Autodesk Inventor part; units mm, degrees
ref_plane "Work Plane1" through (0, -40, 0) normal (-1, 0, 0) x (0, 0, 1)
ref_plane "Work Plane2" through (-196.6667, -40, 18) normal (1, 0, 0) x (0, 0, -1)
ref_plane "YZ Plane" through (0, 0, 0) normal (1, 0, 0) x (0, 1, 0)
sketch "Sketch1" plane through (0, 0, 0) normal (0, 0, 1) x (1, 0, 0)
  line L0 (-590, 40) -> (590, 40)
  line L1 (590, 40) -> (590, -40)
  line L2 (590, -40) -> (-590, -40)
  line L3 (-590, -40) -> (-590, 40)
  point P0 (0, 0)
  point P1 (-590, 0)
  point P2 (0, 40)
  dimension "d0" = 80
  dimension "d1" = 1180
extrude "Extrusion1" add sketch "Sketch1" along normal blind 18
sketch "Sketch2" plane through (0, 0, 18) normal (0, 0, 1) x (1, 0, 0)
  line L0 (590, 40) -> (-590, 40)
  line L1 (-590, 40) -> (-590, -40)
  line L2 (-590, -40) -> (590, -40)
  line L3 (590, -40) -> (590, 40)
  line L4 (-590, 58) -> (-531, 58)
  line L5 (-531, 58) -> (-531, 40)
  line L6 (-531, 40) -> (-590, 40)
  line L7 (-590, 40) -> (-590, 58)
  point P0 (0, 0)
  point P1 (-560.5, 40)
  point P2 (0, 40)
  point P3 (-590, 49)
  point P4 (-590, 0)
  dimension "d4" = 18
  dimension "d5" = 59
extrude "Extrusion2" add sketch "Sketch2" against normal blind 18 contours L0 L7 L4 L5
ref_plane "Work Plane1" through (0, -40, 0) normal (-1, 0, 0) x (0, 0, 1)
sketch "Sketch3" plane through (0, 0, 18) normal (0, 0, 1) x (1, 0, 0)
  line L0 (-246.6667, 58) -> (-146.6667, 58)
  line L1 (-146.6667, 58) -> (-146.6667, 40)
  line L2 (-146.6667, 40) -> (-246.6667, 40)
  line L3 (-246.6667, 40) -> (-246.6667, 58)
  line L4 (590, 40) -> (-531, 40)
  line L5 (-531, 58) -> (-531, 40)
  line L6 (-590, 58) -> (-531, 58)
  line L7 (-590, -40) -> (-590, 58)
  line L8 (-590, -40) -> (590, -40)
  line L9 (590, -40) -> (590, 40)
  point P0 (0, 0)
  point P1 (-196.6667, 40)
  point P2 (29.5, 40)
  dimension "d8" = 18
  dimension "d9" = 100
  dimension "d10" = 393.3333
extrude "Extrusion3" add sketch "Sketch3" against normal blind 18 contours L0 L1 L2 L3
mirror "Mirror1" about plane through (0, -40, 0) normal (-1, 0, 0) of "Extrusion2", "Extrusion3"
sketch "Sketch4" plane through (0, 0, 18) normal (0, 0, 1) x (1, 0, 0)
  line L0 (531, 40) -> (246.6667, 40)
  line L1 (246.6667, 40) -> (246.6667, 58)
  line L2 (246.6667, 58) -> (146.6667, 58)
  line L3 (146.6667, 58) -> (146.6667, 40)
  line L4 (146.6667, 40) -> (-146.6667, 40)
  line L5 (-146.6667, 58) -> (-146.6667, 40)
  line L6 (-246.6667, 58) -> (-146.6667, 58)
  line L7 (-246.6667, 40) -> (-246.6667, 58)
  line L8 (-246.6667, 40) -> (-531, 40)
  line L9 (-531, 58) -> (-531, 40)
  line L10 (-590, 58) -> (-531, 58)
  line L11 (-590, -40) -> (-590, 58)
  line L12 (-590, -40) -> (590, -40)
  line L13 (590, -40) -> (590, 58)
  line L14 (590, 58) -> (531, 58)
  line L15 (531, 58) -> (531, 40)
  line L16 (-590, 9) -> (-572, 9)
  line L17 (-572, 9) -> (-572, -40)
  line L18 (-572, -40) -> (-590, -40)
  line L19 (-590, -40) -> (-590, 9)
  point P0 (0, 0)
  point P1 (-590, -15.5)
  point P2 (-590, 9)
  point P3 (-581, -40)
  point P4 (0, -40)
  dimension "d13" = 18
  dimension "d14" = 49
extrude "Extrusion4" cut sketch "Sketch4" against normal blind 18 contours L12 L11 L16 L17
mirror "Mirror2" about plane through (0, -40, 0) normal (-1, 0, 0) of "Extrusion4"
sketch "Sketch5" plane through (0, 0, 18) normal (0, 0, 1) x (1, 0, 0)
  line L0 (-205.6667, 9) -> (-187.6667, 9)
  line L1 (-187.6667, 9) -> (-187.6667, -40)
  line L2 (-187.6667, -40) -> (-205.6667, -40)
  line L3 (-205.6667, -40) -> (-205.6667, 9)
  line L4 (572, -40) -> (572, 9)
  line L5 (572, 9) -> (590, 9)
  line L6 (590, 9) -> (590, 58)
  line L7 (590, 58) -> (531, 58)
  line L8 (531, 58) -> (531, 40)
  line L9 (531, 40) -> (246.6667, 40)
  line L10 (246.6667, 40) -> (246.6667, 58)
  line L11 (246.6667, 58) -> (146.6667, 58)
  line L12 (146.6667, 58) -> (146.6667, 40)
  line L13 (146.6667, 40) -> (-146.6667, 40)
  line L14 (-146.6667, 58) -> (-146.6667, 40)
  line L15 (-246.6667, 58) -> (-146.6667, 58)
  line L16 (-246.6667, 40) -> (-246.6667, 58)
  line L17 (-246.6667, 40) -> (-531, 40)
  line L18 (-531, 58) -> (-531, 40)
  line L19 (-590, 58) -> (-531, 58)
  line L20 (-590, 9) -> (-590, 58)
  line L21 (-590, 9) -> (-572, 9)
  line L22 (-572, 9) -> (-572, -40)
  line L23 (-572, -40) -> (572, -40)
  point P0 (0, 0)
  point P1 (-196.6667, -40)
  point P2 (0, -40)
  point P3 (-196.6667, 9)
  point P4 (-196.6667, 58)
  dimension "d17" = 18
  dimension "d18" = 49
extrude "Extrusion5" cut sketch "Sketch5" against normal blind 18 contours L0 L1 L2 L3
mirror "Mirror3" about plane through (0, -40, 0) normal (-1, 0, 0) of "Extrusion5"
sketch "Sketch6" plane through (0, 0, 18) normal (0, 0, 1) x (1, 0, 0)
  line L0 (187.6667, -40) -> (187.6667, 9)
  line L1 (187.6667, 9) -> (205.6667, 9)
  line L2 (205.6667, 9) -> (205.6667, -40)
  line L3 (205.6667, -40) -> (572, -40)
  line L4 (572, -40) -> (572, 9)
  line L5 (572, 9) -> (590, 9)
  line L6 (590, 9) -> (590, 58)
  line L7 (590, 58) -> (531, 58)
  line L8 (531, 58) -> (531, 40)
  line L9 (531, 40) -> (246.6667, 40)
  line L10 (246.6667, 40) -> (246.6667, 58)
  line L11 (246.6667, 58) -> (146.6667, 58)
  line L12 (146.6667, 58) -> (146.6667, 40)
  line L13 (146.6667, 40) -> (-146.6667, 40)
  line L14 (-146.6667, 58) -> (-146.6667, 40)
  line L15 (-246.6667, 58) -> (-146.6667, 58)
  line L16 (-246.6667, 40) -> (-246.6667, 58)
  line L17 (-246.6667, 40) -> (-531, 40)
  line L18 (-531, 58) -> (-531, 40)
  line L19 (-590, 58) -> (-531, 58)
  line L20 (-590, 9) -> (-590, 58)
  line L21 (-590, 9) -> (-572, 9)
  line L22 (-572, 9) -> (-572, -40)
  line L23 (-572, -40) -> (-205.6667, -40)
  line L24 (-205.6667, -40) -> (-205.6667, 9)
  line L25 (-205.6667, 9) -> (-187.6667, 9)
  line L26 (-187.6667, 9) -> (-187.6667, -40)
  line L27 (-187.6667, -40) -> (187.6667, -40)
  point P0 (0, 0)
  point P1 (-527.825, 40)
  point P2 (-572, 5.825)
  dimension "d21" = 3.175
  dimension "d22" = 3.175
hole "Hole1" at (-527.825, 40, 18) at (-572, 5.825, 18) direction (0, 0, -1) diameter 6.35 end through all
mirror "Mirror4" about plane through (0, -40, 0) normal (-1, 0, 0) of "Hole1"
sketch "Sketch7" plane through (0, 0, 18) normal (0, 0, 1) x (1, 0, 0)
  arc A0 (524.65, 40) -> (531, 40) centre (527.825, 40) ccw
  line L0 (524.65, 40) -> (246.6667, 40)
  line L1 (246.6667, 40) -> (246.6667, 58)
  line L2 (246.6667, 58) -> (146.6667, 58)
  line L3 (146.6667, 58) -> (146.6667, 40)
  line L4 (146.6667, 40) -> (-146.6667, 40)
  line L5 (-146.6667, 58) -> (-146.6667, 40)
  line L6 (-246.6667, 58) -> (-146.6667, 58)
  line L7 (-246.6667, 40) -> (-246.6667, 58)
  line L8 (-246.6667, 40) -> (-524.65, 40)
  arc A1 (-531, 40) -> (-524.65, 40) centre (-527.825, 40) ccw
  line L9 (-531, 58) -> (-531, 40)
  line L10 (-590, 58) -> (-531, 58)
  line L11 (-590, 9) -> (-590, 58)
  line L12 (-590, 9) -> (-572, 9)
  arc A2 (-572, 2.65) -> (-572, 9) centre (-572, 5.825) ccw
  line L13 (-572, 2.65) -> (-572, -40)
  line L14 (-572, -40) -> (-205.6667, -40)
  line L15 (-205.6667, -40) -> (-205.6667, 9)
  line L16 (-205.6667, 9) -> (-187.6667, 9)
  line L17 (-187.6667, 9) -> (-187.6667, -40)
  line L18 (-187.6667, -40) -> (187.6667, -40)
  line L19 (187.6667, -40) -> (187.6667, 9)
  line L20 (187.6667, 9) -> (205.6667, 9)
  line L21 (205.6667, 9) -> (205.6667, -40)
  line L22 (205.6667, -40) -> (572, -40)
  line L23 (572, -40) -> (572, 2.65)
  arc A3 (572, 9) -> (572, 2.65) centre (572, 5.825) ccw
  line L24 (572, 9) -> (590, 9)
  line L25 (590, 9) -> (590, 58)
  line L26 (590, 58) -> (531, 58)
  line L27 (531, 58) -> (531, 40)
  point P0 (0, 0)
  point P1 (-249.8417, 40)
  point P2 (-205.6667, 5.825)
  dimension "d30" = 3.175
  dimension "d31" = 3.175
hole "Hole2" at (-249.8417, 40, 18) at (-205.6667, 5.825, 18) direction (0, 0, -1) diameter 6.35 end through all
ref_plane "Work Plane2" through (-196.6667, -40, 18) normal (1, 0, 0) x (0, 0, -1)
mirror "Mirror5" about plane through (-196.6667, -40, 18) normal (1, 0, 0) of "Hole2"
mirror "Mirror6" about plane through (0, -40, 0) normal (-1, 0, 0) of "Hole2", "Mirror5"
fillet "Fillet1" radius 3.175 4 edges at (-205.6667, -40, 9) (-187.6667, -40, 9) (187.6667, -40, 9) (205.6667, -40, 9)
equation "\"d0\" = legTopDepth"
equation "\"d1\" = tableLength"
equation "\"d2\" = plyThickness"
equation "\"d4\" = legTopTabHeight"
equation "\"d5\" = 0.5 * plyThickness + 0.5 * legTabTotalWidth"
equation "\"d6\" = plyThickness"
equation "\"d8\" = legTopTabHeight"
equation "\"d9\" = legTabTotalWidth"
equation "\"d11\" = plyThickness"
equation "\"d13\" = plyThickness"
equation "\"d14\" = legTopSlotDepth"
equation "\"d15\" = plyThickness"
equation "\"d17\" = plyThickness"
equation "\"d18\" = legTopSlotDepth"
equation "\"d19\" = plyThickness"
equation "\"d23\" = millDiameter"
equation "\"d32\" = millDiameter"
equation "\"d39\" = 0.5 * millDiameter"
equation "\"plyThickness\" = 18"
equation "\"legHeight\" = 702"
equation "\"tableLength\" = 1180"
equation "\"legTopDepth\" = 80"
equation "\"millDiameter\" = 6.35"
equation "\"legTopTabHeight\" = 18"
equation "\"legTabTotalWidth\" = 100"
equation "\"legTopSlotDepth\" = 49"
properties part number "longSlat"
Verification items for the finished model (mm, model axes). A direction names the side the tool comes from. Coordinates: 2 decimals unless noted, no trailing zeros. Order: outer loops, then holes, each group sorted by start corner. A loop starts at its lowest first (then second) coordinate and runs counter-clockwise, first axis right, second up. Notation, with made-up numbers: (87, 75.25) - (131, 75.25) arc R4 ccw to (131, 79.25) - close; hole circle Ø8 at (82, 67). An arc over 180 degrees is marked (long way). Return JSON: item names as keys, results as strings.
(1) Section check A-A, the plane y = -23. Record the cut outline in (x, z).
Filled sheet:
{"outline": "(-572, 0) - (-205.67, 0) - (-205.67, 18) - (-572, 18) - close; (-187.67, 0) - (187.67, 0) - (187.67, 18) - (-187.67, 18) - close; (205.67, 0) - (572, 0) - (572, 18) - (205.67, 18) - close"}
(2) Access from +Z, -Z, +X, -X, +Y, -Y to the whole of each face (thin tool, end or side, straight path). Record for faces 1 (the flat face through (205.667, -17, 9)), 2 (the flat face through (-531, 49, 9)), 3 (the flat face through (-581, 9, 9)).
Filled sheet:
{"face 1": "+Z, -Z, -Y", "face 2": "+Z, -Z, +Y", "face 3": "+Z, -Z, -X, -Y"}
(3) Section check B-B, the plane x = 471. Record the cut outline in (y, z).
Filled sheet:
{"outline": "(-40, 0) - (40, 0) - (40, 18) - (-40, 18) - close"}
(4) Thickness scan on line 1 along X through (y, z) = (46, 1); line 2 along X through (y, z) = (-27, 5.5); line 3 along Y through (x, z) = (22, 5.75). Record the ranges inside material, lowest first.
Filled sheet:
{"line 1": "x = -590 to -531, -246.67 to -146.67, 146.67 to 246.67, 531 to 590", "line 2": "x = -572 to -205.67, -187.67 to 187.67, 205.67 to 572", "line 3": "y = -40 to 40"}
(5) Go/stop test with flat-tipped pins: pin 1 (9 mm diameter, centred on y = -9.5, z = 11.5, fed in from -X); pin 2 (9 mm diameter, centred on y = -25, z = 9.5, fed in from +X); pin 3 (5.5 mm diameter, centred on x = 398, z = 9, fed in from +Y); pin 4 (5 mm diameter, centred on x = 301.5, y = 11, fed in from -Z). Record where each tip stops, or that it passes through.
Filled sheet:
{"pin 1": "stops at x = -572", "pin 2": "stops at x = 572", "pin 3": "stops at y = 40", "pin 4": "stops at z = 0"}
